from build123d import *

# Parameters (mm, degrees)
F0_W          = 5.842
F0_H          = 12.7
F0_R          = 3.175
F2_DEPTH      = 3.175
F3_R          = 1.524
F4_DEPTH      = 7.62
F4_DEPTH_BACK = 1.27
F5_DEPTH      = 56.134
F6_R          = 1.524
F7_DEPTH      = 17.78


with BuildPart() as f1:
    # F0 (on Front) → F1 (revolve)
    with BuildSketch(Plane.XZ):
        Polygon((5.842, 12.7), (5.842, 0), (66.294, 0), (66.294, 12.7), (56.134, 12.7), (56.134, 10.16), (10.16, 10.16), (10.16, 12.7), align=None)
        with Locations((2.921, 6.35)):
            Rectangle(F0_W, F0_H)
    revolve(axis=Axis((33.147, 0, 0), (-1, 0, 0)))

    # F3 (on face) → F4 (join, two sides)
    with BuildSketch(Plane.YZ.offset(66.294)) as f4_sk:
        with BuildLine():
            ThreePointArc((-5.08, 11.6397422652), (0, 12.7), (5.08, 11.6397422652))
            Line((5.08, 11.6397422652), (5.08, 15.24))
            Line((5.08, 15.24), (-5.08, 15.24))
            Line((-5.08, 15.24), (-5.08, 11.6397422652))
        make_face()
        with BuildLine():
            ThreePointArc((-5.08, 0), (0, 5.08), (5.08, 0))
            Line((5.08, 0), (5.08, 11.6397422652))
            ThreePointArc((5.08, 11.6397422652), (0, 12.7), (-5.08, 11.6397422652))
            Line((-5.08, 11.6397422652), (-5.08, 0))
        make_face()
        with BuildLine():
            ThreePointArc((-5.08, 0), (0, -5.08), (5.08, 0))
            ThreePointArc((5.08, 0), (0, 5.08), (-5.08, 0))
        make_face()
        Circle(F3_R, mode=Mode.SUBTRACT)
    extrude(amount=F4_DEPTH)
    extrude(f4_sk.sketch, amount=-F4_DEPTH_BACK)

    # F5 (cut, through all): a face of the model
    f5_faces = [f1.faces().sort_by_distance(p)[0] for p in [
        (66.294, 0, 0),
    ]]
    extrude(f5_faces, amount=-F5_DEPTH, mode=Mode.SUBTRACT)


with BuildPart() as f2:
    # F0 (on Front) → F2 (new body, symmetric)
    with BuildSketch(Plane.XZ):
        with BuildLine():
            Line((-0.9398, 0), (0, 0))
            Line((0, 0), (0, 12.7))
            Line((0, 12.7), (5.842, 12.7))
            Line((5.842, 12.7), (5.842, 15.24))
            Line((5.842, 15.24), (-0.508, 15.24))
            Line((-0.508, 15.24), (-10.8806298187, 3.8475430269))
            ThreePointArc((-10.8806298187, 3.8475430269), (-4.5919612295, 5.3297205562), (-0.9398, 0))
        make_face()
        with BuildLine():
            ThreePointArc((-8.1826630726, -5.5069827884), (-3.1957909266, -4.5493385486), (-0.9398, 0))
            ThreePointArc((-0.9398, 0), (-4.5919612295, 5.3297205562), (-10.8806298187, 3.8475430269))
            ThreePointArc((-10.8806298187, 3.8475430269), (-12.1459778134, -1.5837270034), (-8.1826630726, -5.5069827884))
        make_face()
        with Locations((-6.6548, 0)):
            Circle(F0_R, mode=Mode.SUBTRACT)
        with BuildLine():
            Line((5.842, 0), (0, 0))
            Line((0, 0), (-0.9398, 0))
            ThreePointArc((-0.9398, 0), (-3.1957909266, -4.5493385486), (-8.1826630726, -5.5069827884))
            Line((-8.1826630726, -5.5069827884), (5.842, -9.398))
            Line((5.842, -9.398), (5.842, 0))
        make_face()
    extrude(amount=F2_DEPTH, both=True)


with BuildPart() as f7_tool:
    # F6 (on face) → F7 (new body)
    with BuildSketch(Plane.XY.offset(15.24)):
        with Locations((2.667, 0)):
            Circle(F6_R)
    extrude(amount=-F7_DEPTH)


with BuildPart() as f1_1:
    add(f1.part)

    # F7: cut by f7_tool
    add(f7_tool.part, mode=Mode.SUBTRACT)


with BuildPart() as f2_1:
    add(f2.part)

    # F7: cut by f7_tool
    add(f7_tool.part, mode=Mode.SUBTRACT)


solid = f1_1.part
The model under review builds one solid part; all positions refer to its coordinate system, in mm. A direction names the side the tool comes from. Give positions to 0.01 mm unless a question says otherwise; leave off trailing zeros. Order: outer loops, then holes, each group sorted by start corner. A loop starts at its lowest first (then second) coordinate and runs counter-clockwise, first axis right, second up. Notation, with made-up numbers: M 74,36 L 96,36 A20 ccw 96,74 Z; hole C 44,23 d2. An arc over 180 degrees is marked long. Answer in a Markdown table with one row per item. Add a question column.
1. Add section D-D on z = -7.75. State the section outline as (x, y) points, plus the area to 3 significant figures.
2. Add section C-C on y = 0. State the section outline as (x, z) points.
3. Mouldability with a two-part tool opening along Y and no side actions: class faces 5 (the flat face through (70, 0, 15.24)), 6 (the cylindrical face through (70.05, -0.11, -5.08)), 7 (the flat face through (70, -5.08, 8)), 8 (the flat face through (3, 0, -2.54)) as released by +Y, released by -Y, zero draft, split by the parting line, or undercut.
4. To check wall thickness, follow line 1 along X through (y, z) = (-6.5, -8.25); line 2 along X through (y, z) = (0, 1.25); line 3 along X through (y, z) = (4.5, -5.25). State the ranges of each line that lie inside material, in increasing order.
5. Add section B-B on x = 42.5. State the section outline as (y, z) points, plus the area to 3 significant figures.
6. Add section A-A on z = 4.75. State the section outline as (x, y) points, plus the area to 3 significant figures.
7. Machinability: for faces 1 (the cylindrical face through (61.143, 0.558, -12.688)), 2 (the cylindrical face through (41.59, -0.2, 1.51)), 3 (the cylindrical face through (32.825, 10.074, -1.323)), 4 (the flat face through (66.294, 0, -6)), which of the approach directions +Z, -Z, +X, -X, +Y, -Y give a long, thin tool a straight path to every point of the face, cutting with its end or side? Answer none if there is none.
8. For pin 1 Ø8 at (x, z) = (33, -4) entering from -Y; pin 2 Ø8 at (x, z) = (64, 6.5) entering from +Y; pin 3 Ø2 at (x, z) = (45, 3) entering from +Y, all flat-tipped, find the tip position at first contact; note any pin that passes through.
The answers:
| question | item | result |
|---|---|---|
| 1 | outline | M 0,-10.06 L 10.16,-10.06 L 10.16,-6.57 L 56.13,-6.57 L 56.13,-10.06 L 66.29,-10.06 L 66.29,10.06 L 56.13,10.06 L 56.13,6.57 L 10.16,6.57 L 10.16,10.06 L 0,10.06 Z |
| 1 | area | 1,010 mm2 |
| 2 | outline | M 0,-12.7 L 10.16,-12.7 L 10.16,-10.16 L 56.13,-10.16 L 56.13,-12.7 L 66.29,-12.7 L 66.29,-5.08 L 73.91,-5.08 L 73.91,-1.52 L 10.16,-1.52 L 10.16,1.52 L 73.91,1.52 L 73.91,15.24 L 65.02,15.24 L 65.02,12.7 L 56.13,12.7 L 56.13,10.16 L 10.16,10.16 L 10.16,12.7 L 4.19,12.7 L 4.19,-2.54 L 1.14,-2.54 L 1.14,12.7 L 0,12.7 Z |
| 3 | face 5 | zero draft |
| 3 | face 6 | split by the parting line |
| 3 | face 7 | released by -Y |
| 3 | face 8 | undercut |
| 4 | line 1 | 0 to 10.16, 56.13 to 66.29 |
| 4 | line 2 | 0 to 1.14, 4.19 to 10.16 |
| 4 | line 3 | 0 to 66.29 |
| 5 | outline | C 0,0 d20.32; hole C 0,0 d3.05 |
| 5 | area | 317 mm2 |
| 6 | outline | M 0,-11.78 L 10.16,-11.78 L 10.16,-8.98 L 56.13,-8.98 L 56.13,-11.78 L 66.29,-11.78 L 66.29,-5.08 L 73.91,-5.08 L 73.91,5.08 L 66.29,5.08 L 66.29,11.78 L 56.13,11.78 L 56.13,8.98 L 10.16,8.98 L 10.16,11.78 L 0,11.78 Z; hole C 2.67,0 d3.05 |
| 6 | area | 1,370 mm2 |
| 7 | face 1 | -X |
| 7 | face 2 | +X |
| 7 | face 3 | none |
| 7 | face 4 | -Z, +X |
| 8 | pin 1 | y = -10.16 |
| 8 | pin 2 | y = 12.45 |
| 8 | pin 3 | y = 9.96 |
